Could you check a few things on this drawing? It's one solid part, dimensions in mm from its lowest x, y, z. Round coordinates to 2 decimals unless told otherwise and drop trailing zeros. Order: outer loops, then holes, each group sorted by start corner. A loop starts at its lowest first (then second) coordinate and runs counter-clockwise, first axis right, second up.
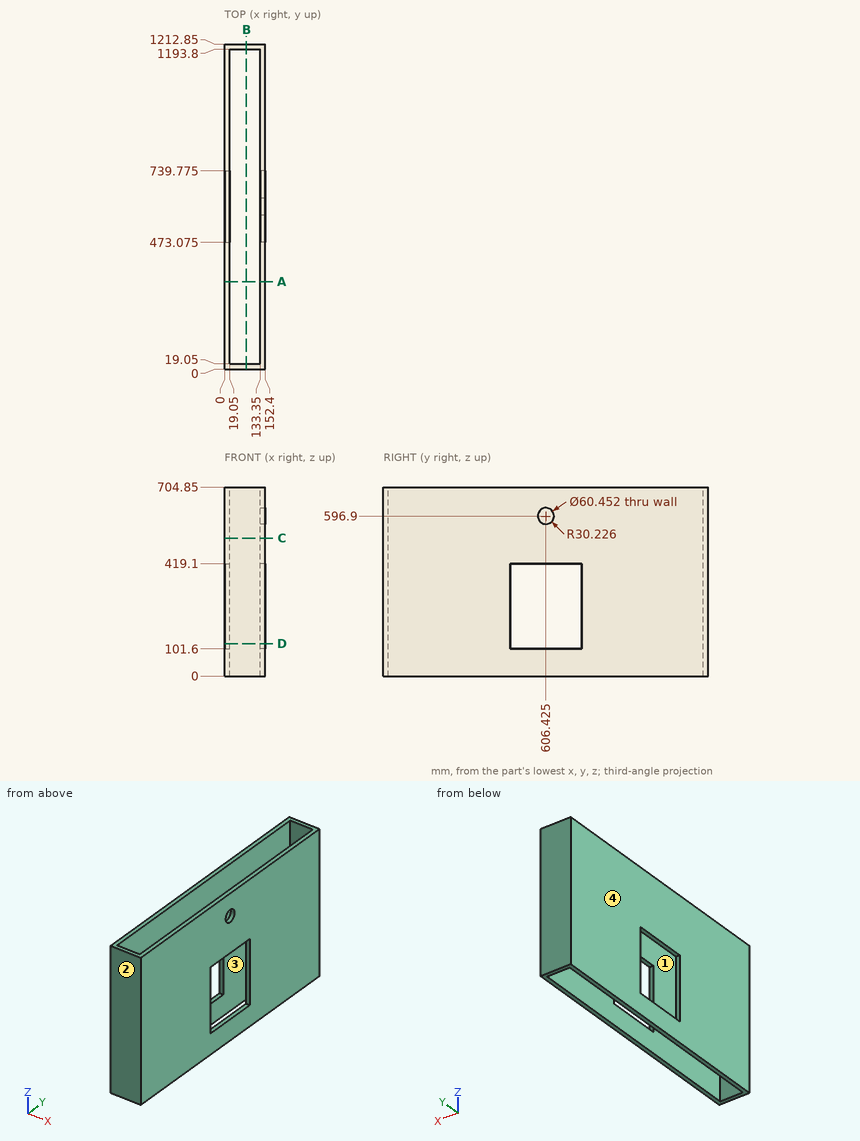
(1) If we mould it in two halves opening along Y, with no side actions, what happens to the marked faces 1, 2, 3 and 4? For each: pulls with the +Y half, pulls with the -Y half, needs draft (parallel to the pull), parting line crosses it, or undercut.
(2) I want a section at A-A, the plane y = 326. List the corners of the cut face in (x, z) for me, plus the area to 3 significant figures.
(3) I want a section at D-D, the plane z = 120.5. List the corners of the cut face in (x, y) for me (3 decimals), plus the area to 3 significant figures.
(4) I'm going to push flat-ended pins straight in: pin 1 Ø4 at (x, y) = (133, 890) entering from -Z; pin 2 Ø12 at (x, y) = (122, 964.5) entering from +Z. Where does each tip first touch, or does it pass through?
(5) I want a section at B-B, the plane x = 81.5. List the corners of the cut face in (y, z) for me.
(6) I want a section at C-C, the plane z = 514. List the corners of the cut face in (x, y) for me, plus the area to 3 significant figures.
(7) Please list where these lines run through material, in increasing order: probe 1 along X at (y, z) = (534, 514.5); probe 2 along Y at (x, z) = (98, 672).
Ans:
1. face 1: undercut
1. face 2: pulls with the -Y half
1. face 3: undercut
1. face 4: needs draft
2. outline: (0, 0) - (19.05, 0) - (19.05, 704.85) - (0, 704.85) - close; (133.35, 0) - (152.4, 0) - (152.4, 704.85) - (133.35, 704.85) - close
2. area: 26,900 mm2
3. outline: (0, 0) - (152.4, 0) - (152.4, 473.075) - (133.35, 473.075) - (133.35, 19.05) - (19.05, 19.05) - (19.05, 473.075) - (0, 473.075) - close; (0, 739.775) - (19.05, 739.775) - (19.05, 1193.8) - (133.35, 1193.8) - (133.35, 739.775) - (152.4, 739.775) - (152.4, 1212.85) - (0, 1212.85) - close
3. area: 40,400 mm2
4. pin 1: stops at z = 0
4. pin 2: passes through
5. outline: (0, 0) - (19.05, 0) - (19.05, 704.85) - (0, 704.85) - close; (1193.8, 0) - (1212.85, 0) - (1212.85, 704.85) - (1193.8, 704.85) - close
6. outline: (0, 0) - (152.4, 0) - (152.4, 1212.85) - (0, 1212.85) - close; hole (19.05, 19.05) - (133.35, 19.05) - (133.35, 1193.8) - (19.05, 1193.8) - close
6. area: 50,600 mm2
7. probe 1: x = 0 to 19.05, 133.35 to 152.4
7. probe 2: y = 0 to 19.05, 1193.8 to 1212.85
